Could you check a few things on this model? Use its own coordinates, in mm. Face numbers are marked on the shaded views. Give positions to 0.01 mm unless a question says otherwise; leave off trailing zeros. Loops run counter-clockwise (first coordinate to the right, second up) from the corner with the lowest first, then second, coordinate; pieces in that order, holes last. Notation, with made-up numbers: (50, 28) - (94, 28) arc R34 ccw to (94, 62) - close; hole circle Ø5 at (-2.75, 62.25). An arc over 180 degrees is marked (long way). Use CSV: the item, a comma, the result in double quotes.
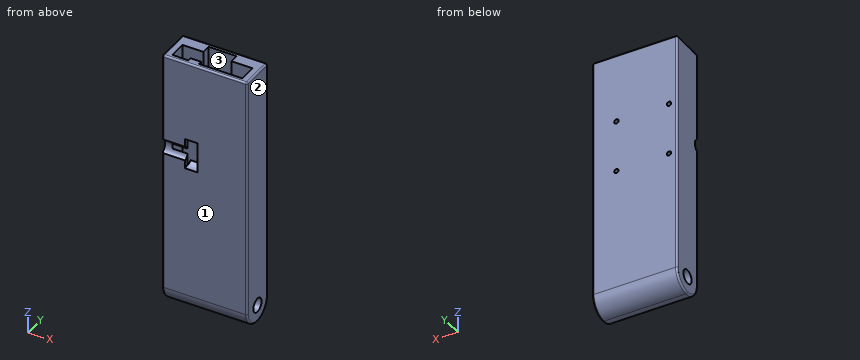
from build123d import *

# Parameters (mm, degrees)
SKETCH_1_W               = 48.5
SKETCH_1_H               = 150
EXTRUDE_1_DEPTH          = 20
CUT_EXTRUDE_1_REACH      = 93.527
CUT_EXTRUDE_2_REACH      = 93.527
SKETCH_4_R               = 4
M3X0_5_1_D               = 2.5
M3X0_5_1_DEPTH           = 7.5
M3X0_5_1_TIP             = 0.751075774
CUT_EXTRUDE_3_DEPTH      = 14
CUT_EXTRUDE_4_DEPTH      = 1
CUT_EXTRUDE_4_DEPTH_BACK = 6
CUT_EXTRUDE_5_DEPTH      = 120
FILLET_1_R               = 1


with BuildPart() as part:
    # 草图1 → 凸台-拉伸1 (new body)
    with BuildSketch(Plane(origin=(0, 0, 0), x_dir=(1, 0, 0), z_dir=(0, 1, 0))):
        Rectangle(SKETCH_1_W, SKETCH_1_H)
    extrude(amount=EXTRUDE_1_DEPTH)

    # 草图3 → 切除-拉伸1 (cut, up to next)
    with BuildSketch(Plane(origin=(24.25, 0, 0), x_dir=(0, 0, -1), z_dir=(1, 0, 0)), mode=Mode.PRIVATE) as cut_extrude_1_sk1:
        with BuildLine():
            Line((75, 0), (75, 10))
            ThreePointArc((75, 10), (72.071067812, 2.928932188), (65, 0))
            Line((65, 0), (75, 0))
        make_face()
    cut_extrude_1_tool1 = extrude(cut_extrude_1_sk1.sketch, amount=-CUT_EXTRUDE_1_REACH, mode=Mode.PRIVATE) & part.part
    # 草图3 → 切除-拉伸1 (cut, up to next)
    with BuildSketch(Plane(origin=(24.25, 0, 0), x_dir=(0, 0, -1), z_dir=(1, 0, 0)), mode=Mode.PRIVATE) as cut_extrude_1_sk2:
        with BuildLine():
            Line((75, 20), (65, 20))
            ThreePointArc((65, 20), (72.071067812, 17.071067812), (75, 10))
            Line((75, 10), (75, 20))
        make_face()
    cut_extrude_1_tool2 = extrude(cut_extrude_1_sk2.sketch, amount=-CUT_EXTRUDE_1_REACH, mode=Mode.PRIVATE) & part.part
    add(cut_extrude_1_tool1.solids().sort_by_distance((24.25, 2.233679, -72.766321))[0], mode=Mode.SUBTRACT)
    add(cut_extrude_1_tool2.solids().sort_by_distance((24.25, 17.766321, -72.766321))[0], mode=Mode.SUBTRACT)

    # 草图4 → 切除-拉伸2 (cut, up to next)
    with BuildSketch(Plane(origin=(24.25, 0, 0), x_dir=(0, 0, -1), z_dir=(1, 0, 0)), mode=Mode.PRIVATE) as cut_extrude_2_sk1:
        with Locations((65, 10)):
            Circle(SKETCH_4_R)
    cut_extrude_2_tool1 = extrude(cut_extrude_2_sk1.sketch, amount=-CUT_EXTRUDE_2_REACH, mode=Mode.PRIVATE) & part.part
    add(cut_extrude_2_tool1.solids().sort_by_distance((24.25, 10, -65))[0], mode=Mode.SUBTRACT)

    # M3x0.5 螺纹孔1
    with Locations(Plane(origin=(-19.5, 20, 5), x_dir=(0, 0, 1), z_dir=(0, 1, 0))):
        with Locations((0, 0), (0, 30), (30, 0), (30, 30)):
            Hole(M3X0_5_1_D / 2, depth=M3X0_5_1_DEPTH)
            with Locations((0, 0, -(M3X0_5_1_DEPTH + M3X0_5_1_TIP / 2))):  # 118° drill point
                Cone(0, M3X0_5_1_D / 2, M3X0_5_1_TIP, mode=Mode.SUBTRACT)

    # 草图9 → 切除-拉伸3 (cut)
    with BuildSketch(Plane.ZY.offset(24.25)):
        with BuildLine():
            Line((24.145780988, 0), (15.854219012, 0))
            ThreePointArc((15.854219012, 0), (20, 2.75), (24.145780988, 0))
        make_face()
    extrude(amount=-CUT_EXTRUDE_3_DEPTH, mode=Mode.SUBTRACT)

    # 草图10 → 切除-拉伸4 (cut, two sides: drawn at the far end of the back side and taken through both)
    with BuildSketch(Plane.ZY.offset(10.25).offset(-CUT_EXTRUDE_4_DEPTH_BACK)):
        with BuildLine():
            Line((28.828221792, 0), (11.171778209, 0))
            ThreePointArc((11.171778209, 0), (20, 7.25), (28.828221792, 0))
        make_face()
    extrude(amount=CUT_EXTRUDE_4_DEPTH + CUT_EXTRUDE_4_DEPTH_BACK, mode=Mode.SUBTRACT)

    # 草图11 → 切除-拉伸5 (cut)
    with BuildSketch(Plane.XY.offset(75)):
        Polygon((-4.7499492, 2.5), (20, 2.5), (20, 12.5), (8, 12.5), (8, 17.5), (-8, 17.5), (-8, 12.5), (-20, 12.5), (-20, 2.5), (-10.7499492, 2.5), (-10.7499492, 4.5), (-4.7499492, 4.5), align=None)
    extrude(amount=-CUT_EXTRUDE_5_DEPTH, mode=Mode.SUBTRACT)

    # 圆角1
    fillet_1_edges = [part.edges().sort_by_distance(p)[0] for p in [
        (-24.25, 0, -24.572890494),
        (0, 20, 75),
        (24.25, 10, -75),
        (-24.25, 10, -75),
        (-24.25, 20, 5),
        (24.25, 20, 5),
        (0, 0, 75),
        (-24.25, 0, 49.572890494),
        (24.25, 0, 5),
        (24.25, 10, 75),
        (-24.25, 10, 75),
    ]]
    fillet(fillet_1_edges, radius=FILLET_1_R)


solid = part.part
1) Suppose I cut it at A-A (z = -19). Please give me the cut outline in (x, y), plus the area to 3 significant figures.
Answer below:
outline,"(-24.25, 1) arc R1 ccw to (-23.25, 0) - (23.25, 0) arc R1 ccw to (24.25, 1) - (24.25, 19) arc R1 ccw to (23.25, 20) - (-23.25, 20) arc R1 ccw to (-24.25, 19) - close; hole (-20, 2.5) - (-10.75, 2.5) - (-10.75, 4.5) - (-4.75, 4.5) - (-4.75, 2.5) - (20, 2.5) - (20, 12.5) - (8, 12.5) - (8, 17.5) - (-8, 17.5) - (-8, 12.5) - (-20, 12.5) - close"
area,"501 mm2"
2) We'd pull the mould along X, two halves only. Please class the marked faces 1, 2 and 3: +X half, -X half, draft (parallel to the pull), parting line (faces both ways), or undercut.
Answer below:
face 1,"draft"
face 2,"+X half"
face 3,"undercut"
3) I'm going to push flat-ended pins straight in: P1, Ø4.5, axis at x = -6.5, y = 7, coming from the +Z side; P2, Ø1.5, axis at x = -13, y = 16.5, coming from the -Z side. Where does each tip first touch, or does it pass through?
Answer below:
P1,"stops at z = -45"
P2,"stops at z = -73.18"
4) I need wall thicknesses on line 1 along X through (y, z) = (17.25, 5); line 2 along Y through (x, z) = (2, 24.5); line 3 along Y through (x, z) = (-16, 57). Which ranges of each line are inside material? Lowest first, please.
Answer below:
line 1,"x = -24.25 to -20.75, -18.25 to -8, 8 to 9.25, 11.75 to 24.25"
line 2,"y = 0 to 2.5, 17.5 to 20"
line 3,"y = 0 to 2.5, 12.5 to 20"
